Autodesk Inventor part; units mm, degrees
ref_plane "YZ Plane" through (0, 0, 0) normal (1, 0, 0) x (0, 1, 0)
ref_plane "XZ Plane" through (0, 0, 0) normal (0, 1, 0) x (-1, 0, 0)
ref_plane "XY Plane" through (0, 0, 0) normal (0, 0, 1) x (1, 0, 0)
sketch "草图1" plane through (0, 0, 0) normal (0, 0, 1) x (1, 0, 0)
  circle A0 centre (0, 0) radius 28
  circle A1 centre (0, 0) radius 7.5
  dimension "d0" = 56
  dimension "d1" = 15
extrude "拉伸1" add sketch "草图1" along normal blind 9
sketch "草图2" plane through (0, 0, 9) normal (0, 0, 1) x (1, 0, 0)
  circle A0 centre (0, 0) radius 28
  circle A1 centre (0, 0) radius 7.5
  dimension "d4" = 15
extrude "拉伸2" add sketch "草图2" along normal blind 2
sketch "草图3" plane through (0, 0, 11) normal (0, 0, 1) x (1, 0, 0)
  circle A0 centre (0, 0) radius 14.5 construction
  line L0 (-36.9419, 0) -> (43.6936, 0) construction
  circle A1 centre (14.5, 0) radius 1.6
  circle A2 centre (10.253, 10.253) radius 1.6
  circle A3 centre (0, 14.5) radius 1.6
  circle A4 centre (-10.253, 10.253) radius 1.6
  circle A5 centre (-14.5, 0) radius 1.6
  circle A6 centre (-10.253, -10.253) radius 1.6
  circle A7 centre (0, -14.5) radius 1.6
  circle A8 centre (10.253, -10.253) radius 1.6
  dimension "d7" = 29
  dimension "d8" = 3.2
  dimension "d11" = 360
extrude "拉伸3" cut sketch "草图3" against normal through all
chamfer "倒角1" distance 1 angle 45 2 edges at (-28, 0, 0) (-28, 0, 11)
sketch "草图4" plane through (0, 0, 0) normal (0, 0, -1) x (-1, 0, 0)
  circle A0 centre (0, 0) radius 18.5
  circle A1 centre (0, 0) radius 23
  dimension "d18" = 37
  dimension "d19" = 46
extrude "拉伸4" cut sketch "草图4" against normal blind 2
sketch "草图6" plane through (0, 0, 0) normal (0, 0, -1) x (-1, 0, 0)
  circle A0 centre (0, 0) radius 18.5
  circle A1 centre (0, 0) radius 7.5
  circle A2 centre (-14.5, 0) radius 1.6
  circle A3 centre (-10.253, 10.253) radius 1.6
  circle A4 centre (0, 14.5) radius 1.6
  circle A5 centre (10.253, 10.253) radius 1.6
  circle A6 centre (14.5, 0) radius 1.6
  circle A7 centre (10.253, -10.253) radius 1.6
  circle A8 centre (0, -14.5) radius 1.6
  circle A9 centre (-10.253, -10.253) radius 1.6
extrude "拉伸6" add sketch "草图6" along normal blind 4
sketch "草图7" plane through (0, 0, 11) normal (0, 0, 1) x (1, 0, 0)
  circle A0 centre (0, 0) radius 20
  circle A1 centre (0, 0) radius 7.5
  dimension "d34" = 40
extrude "拉伸7" cut sketch "草图7" against normal blind 4
chamfer "倒角3" distance 1 angle 45 2 edges at (-20, 0, 11) (-20, 0, 7)
properties part number "内轮"
Input: part model. Units: mm. Frame: model coordinates. A direction names the side the tool comes from. Give positions to 0.01 mm unless a question says otherwise; leave off trailing zeros. Order: outer loops, then holes, each group sorted by start corner. A loop starts at its lowest first (then second) coordinate and runs counter-clockwise, first axis right, second up. Notation, with made-up numbers: (67, -33) -> (84, -33) arc R24 cw to (84, -9) -> close; hole circle Ø2 at (29, -13.75). An arc over 180 degrees is marked (long way). Use one line per item in the form item = value.
1) Section D-D, the plane z = 9. Return loops of the section in (x, y), and give its area (3 significant figures).
Response values:
outline = circle Ø56 at (0, 0); hole circle Ø40 at (0, 0)
area = 1,210 mm^2
2) Reachability of faces 1 (the flat face through (-2, 19, 2)), 2 (the cylindrical face through (-10.15, 11.85, 1.58)), 3 (the flat face through (0, -8, 7)) from +Z, -Z, +X, -X, +Y, -Y: full face, straight path, thin tool, end or side. Return the list, or none.
Response values:
face_1 = -Z
face_2 = +Z, -Z
face_3 = +Z
3) First-contact query: pin 1 Ø1.5 at (y, z) = (13.5, 6) entering from -X; pin 2 Ø2 at (y, z) = (9.5, 8) entering from +X; pin 3 Ø1 at (x, z) = (-21.5, 9) entering from +Y; pin 4 Ø1.9 at (x, y) = (-10.253, -10.253) entering from -Z. Flat tips, straight axial feed; report the tip coordinate or a pass-through.
Response values:
pin_1 = -24.93
pin_2 = 26.68
pin_3 = 18.52
pin_4 = through
4) Section A-A, the plane z = -1.25. Count the separate pieces of the cut face and the enclosed holes in it, and give its area (3 significant figures).
Response values:
separate_pieces = 1
enclosed_holes = 9
area = 834 mm^2
5) Mould query, pull axis X, two halves, no side actions, for faces 4 (the cylindrical face through (0.105, -12.903, 1.577)), 5 (the flat face through (-8, 0, -4)), 6 (the cylindrical face through (-14.395, 1.597, 1.577)), 7 (the cylindrical face through (25.865, 10.724, 5.437)). Classes: pulls with the +X half, pulls with the -X half, needs draft (parallel to the pull), parting line crosses it, or undercut.
Response values:
face_4 = undercut
face_5 = needs draft
face_6 = undercut
face_7 = parting line crosses it
6) Line query: probe 1 along Y at (x, z) = (0, -1); probe 2 along Y at (x, z) = (-14.5, 0.5); probe 3 along X at (y, z) = (14, 1). Output: solid intervals per line, ascending.
Response values:
probe_1 = -18.5 to -16.1, -12.9 to -7.5, 7.5 to 12.9, 16.1 to 18.5
probe_2 = -23.37 to -17.85, -11.49 to -1.6, 1.6 to 11.49, 17.85 to 23.37
probe_3 = -24.25 to -18.25, -12.09 to -1.52, 1.52 to 12.09, 18.25 to 24.25
